from build123d import *

# Parameters (mm, degrees)
F0_W     = 366
F0_H     = 55
F1_DEPTH = 19
F2_W     = 8
F2_H     = 55
F2_W_2   = 3
F3_DEPTH = 8
F4_W     = 8
F4_H     = 55
F4_W_2   = 3
F5_DEPTH = 8


with BuildPart() as f1:
    # F0 (on Front) → F1 (new body)
    with BuildSketch(Plane.XZ):
        Rectangle(F0_W, F0_H)
    extrude(amount=F1_DEPTH)

    # F2 (on face) → F3 (cut)
    with BuildSketch(Plane.YZ.offset(183)):
        with Locations((-15, 0)):
            Rectangle(F2_W, F2_H)
        with Locations((-1.5, 0)):
            Rectangle(F2_W_2, F2_H)
    extrude(amount=-F3_DEPTH, mode=Mode.SUBTRACT)

    # F4 (on face) → F5 (cut)
    with BuildSketch(Plane(origin=(-183, 0, 0), x_dir=(0, -1, 0), z_dir=(-1, 0, 0))):
        with Locations((15, 0)):
            Rectangle(F4_W, F4_H)
        with Locations((1.5, 0)):
            Rectangle(F4_W_2, F4_H)
    extrude(amount=-F5_DEPTH, mode=Mode.SUBTRACT)


solid = f1.part
Geometry: final body of the model. Coordinates: model frame, mm. A direction names the side the tool comes from. Coordinates: 2 decimals unless noted, no trailing zeros. Loops run counter-clockwise (first coordinate to the right, second up) from the corner with the lowest first, then second, coordinate; pieces in that order, holes last. Notation, with made-up numbers: (86, 42.5) - (126, 42.5) arc R26 ccw to (126, 71.5) - close; hole circle Ø10 at (3.5, 62). An arc over 180 degrees is marked (long way). One line per question, with ' | ' between items. Start each with the question number.
(1) Ray query, L1, parallel to X at y = -0.75, z = 0. Return the intervals inside material, ascending. Write a range as from..to.
(2) Cut plane A-A on z = 15. Output: boundary loops of the cut face in (x, y), and give its area (3 significant figures).
(3) First-contact query: pin 1 (4 mm diameter, centred on x = 177.5, z = 11, fed in from +Y); pin 2 (2.5 mm diameter, centred on x = 181, z = 5, fed in from -Y); pin 3 (9 mm diameter, centred on y = -16.5, z = -1, fed in from +X). Flat tips, straight axial feed; report the tip coordinate or a pass-through.
(4) Cut plane B-B on y = -15.5. Output: boundary loops of the cut face in (x, z), and give its area (4 significant figures).
(5) Reachability of faces 1 (the flat face through (179, -11, 0)), 2 (the flat face through (179, -3, 0)), 3 (the flat face through (-179, -3, 0)), 4 (the flat face through (-179, -11, 0)) from +Z, -Z, +X, -X, +Y, -Y: full face, straight path, thin tool, end or side. Return the list, or none.
Here are the results:
1) L1: -175..175
2) outline: (-183, -11) - (-175, -11) - (-175, -19) - (175, -19) - (175, -11) - (183, -11) - (183, -3) - (175, -3) - (175, 0) - (-175, 0) - (-175, -3) - (-183, -3) - close | area: 6,780 mm²
3) pin 1: y = -3 | pin 2: y = -11 | pin 3: x = 175
4) outline: (-175, -27.5) - (175, -27.5) - (175, 27.5) - (-175, 27.5) - close | area: 19,250 mm²
5) face 1: +Z, -Z, +X, -Y | face 2: +Z, -Z, +X, +Y | face 3: +Z, -Z, -X, +Y | face 4: +Z, -Z, -X, -Y
